Source: CAD feature listing. Evaluate the final solid. Frame: model axes, mm. Face numbers are marked on the shaded views. A direction names the side the tool comes from. Give positions to 0.01 mm unless a question says otherwise; leave off trailing zeros. Order: outer loops, then holes, each group sorted by start corner. A loop starts at its lowest first (then second) coordinate and runs counter-clockwise, first axis right, second up.
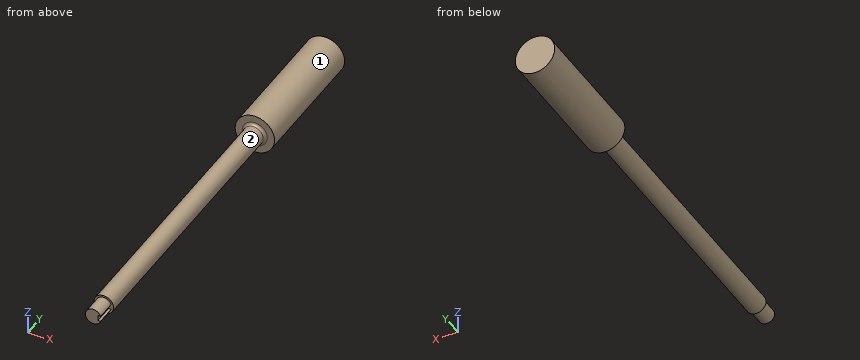
from build123d import *

# Parameters (mm, degrees)
SKETCH1_R           = 7.5
BOSS_EXTRUDE1_DEPTH = 215.44
SKETCH5_R           = 15
BOSS_EXTRUDE5_DEPTH = 5
SKETCH6_R           = 15
SKETCH6_R_2         = 12.5
BOSS_EXTRUDE6_DEPTH = 90
SKETCH7_R           = 15
BOSS_EXTRUDE7_DEPTH = 5
FILLET2_R           = 2
SKETCH9_R           = 6
BOSS_EXTRUDE9_DEPTH = 15
SKETCH12_W          = 15.293303155
SKETCH12_H          = 4
CUT_EXTRUDE3_DEPTH  = 15


with BuildPart() as part:
    # Sketch1 → Boss-Extrude1 (new body)
    with BuildSketch(Plane(origin=(0, 0, 0), x_dir=(1, 0, 0), z_dir=(0, 1, 0))):
        with Locations(Location((0, 0, 0), (0, 0, 270))):
            Circle(SKETCH1_R)
    extrude(amount=BOSS_EXTRUDE1_DEPTH)

    # Sketch5 → Boss-Extrude5 (add)
    with BuildSketch(Plane(origin=(0, 215.44, 0), x_dir=(1, 0, 0), z_dir=(0, 1, 0))):
        with Locations(Location((0, 0, 0), (0, 0, 270))):
            Circle(SKETCH5_R)
    extrude(amount=BOSS_EXTRUDE5_DEPTH)

    # Sketch6 → Boss-Extrude6 (add)
    with BuildSketch(Plane(origin=(0, 220.44, 0), x_dir=(1, 0, 0), z_dir=(0, 1, 0))):
        with Locations(Location((0, 0, 0), (0, 0, 270))):
            Circle(SKETCH6_R)
        with Locations(Location((0, 0, 0), (0, 0, 90))):
            Circle(SKETCH6_R_2, mode=Mode.SUBTRACT)
    extrude(amount=BOSS_EXTRUDE6_DEPTH)

    # Sketch7 → Boss-Extrude7 (add)
    with BuildSketch(Plane(origin=(0, 310.44, 0), x_dir=(1, 0, 0), z_dir=(0, 1, 0))):
        with Locations(Location((0, 0, 0), (0, 0, 270))):
            Circle(SKETCH7_R)
    extrude(amount=BOSS_EXTRUDE7_DEPTH)

    # Fillet2
    fillet2_edges = [part.edges().sort_by_distance(p)[0] for p in [
        (0, 215.44, -7.5),
    ]]
    fillet(fillet2_edges, radius=FILLET2_R)

    # Sketch9 → Boss-Extrude9 (add)
    with BuildSketch(Plane.XZ):
        with Locations(Location((0, 0, 0), (0, 0, 90))):
            Circle(SKETCH9_R)
    extrude(amount=BOSS_EXTRUDE9_DEPTH)

    # Sketch12 → Cut-Extrude3 (cut)
    with BuildSketch(Plane.XZ.offset(15)):
        with Locations((11.306651578, 0)):
            Rectangle(SKETCH12_W, SKETCH12_H)
    extrude(amount=-CUT_EXTRUDE3_DEPTH, mode=Mode.SUBTRACT)


solid = part.part
1) Section query C-C on y = 67. Output: boundary loops of the cut face in (x, z), and give its area (3 significant figures).
Checks:
outline: circle Ø15 at (0, 0)
area: 177 mm2
2) First-contact query: pin 1 Ø0.6 at (x, y) = (5, -9.5) entering from -Z; pin 2 Ø1.2 at (y, z) = (-5.5, 1) entering from +X; pin 3 Ø2 at (x, y) = (4.5, -8.5) entering from +Z. Flat tips, straight axial feed; report the tip coordinate or a pass-through.
Checks:
pin 1: stops at z = -3.73
pin 2: stops at x = 3.66
pin 3: stops at z = 4.87
3) Ray query, L1, parallel to Y at x = -12, z = -3; L2, parallel to Z at x = -0.5, y = 274.5; L3, parallel to X at y = 285, z = 0. Return the intervals inside material, ascending.
Checks:
L1: y = 215.44 to 220.44, 310.44 to 315.44
L2: z = -14.99 to -12.49, 12.49 to 14.99
L3: x = -15 to -12.5, 12.5 to 15
4) Section query A-A on x = 0. Output: boundary loops of the cut face in (y, z), and give its area (3 significant figures).
Checks:
outline: (-15, -6) - (0, -6) - (0, -7.5) - (213.44, -7.5) arc R2 cw to (215.44, -9.5) - (215.44, -15) - (315.44, -15) - (315.44, 15) - (215.44, 15) - (215.44, 9.5) arc R2 cw to (213.44, 7.5) - (0, 7.5) - (0, 6) - (-15, 6) - close; hole (220.44, -12.5) - (310.44, -12.5) - (310.44, 12.5) - (220.44, 12.5) - close
area: 4,160 mm2
5) Section query B-B on y = 246. Output: boundary loops of the cut face in (x, z), and give its area (3 significant figures).
Checks:
outline: circle Ø30 at (0, 0); hole circle Ø25 at (0, 0)
area: 216 mm2
6) Reachability of the marked faces 1 and 2 from +Z, -Z, +X, -X, +Y, -Y: full face, straight path, thin tool, end or side. Return the list, or none.
Checks:
face 1: +Y, -Y
face 2: -Y
